```python
from build123d import *

# Parameters (mm, degrees)
F2_DEPTH = 6.35
F1_W     = 1.778
F1_H     = 3.048
F1_H_2   = 5.842
F1_W_2   = 0.762
F5_DEPTH = 12.7
F6_DEPTH = 2.54


# Not quite as in the source:
# - a feature names something its author has since deleted; it is built from what else it names


with BuildPart() as f2:
    # F0 (on Top) → F2 (new body)
    with BuildSketch(Plane.XY):
        with BuildLine():
            ThreePointArc((-19.5801208863, -2.5399817128), (-19.1839428746, -1.2973564714), (-19.05, 0))
            ThreePointArc((-19.05, 0), (-19.1839428746, 1.2973564714), (-19.5801208863, 2.5399817128))
            ThreePointArc((-19.5801208863, 2.5399817128), (-21.0323461368, 4.6093491657), (-23.1768579109, 5.9481206487))
            ThreePointArc((-23.1768579109, 5.9481206487), (-31.75, 0), (-23.1768579109, -5.9481206487))
            ThreePointArc((-23.1768579109, -5.9481206487), (-21.0323461368, -4.6093491657), (-19.5801208863, -2.5399817128))
        make_face()
        with BuildLine():
            ThreePointArc((-23.1768579109, 5.9481206487), (-21.0323461368, 4.6093491657), (-19.5801208863, 2.5399817128))
            add(Edge.make_bspline(
                [(0, 1.524), (-9.0764431036, 1.3546369813), (-12.8672626316, 1.8652065321), (-19.5801208863, 2.5399817128)],
                knots=[0, 0, 0, 0, 19.6064620154, 19.6064620154, 19.6064620154, 19.6064620154], degree=3))
            add(Edge.make_bspline(
                [(0, 1.524), (9.0764431036, 1.3546369813), (12.8672626316, 1.8652065321), (19.5801208863, 2.5399817128)],
                knots=[0, 0, 0, 0, 19.6064620154, 19.6064620154, 19.6064620154, 19.6064620154], degree=3))
            ThreePointArc((19.5801208863, 2.5399817128), (21.0323461368, 4.6093491657), (23.1768579109, 5.9481206487))
            add(Edge.make_bspline(
                [(0, 2.54), (8.1250406802, 3.246476237), (13.1090918084, 2.1852389104), (23.1768579109, 5.9481206487)],
                knots=[0, 0, 0, 0, 23.4260971776, 23.4260971776, 23.4260971776, 23.4260971776], degree=3))
            add(Edge.make_bspline(
                [(0, 2.54), (-8.1250406802, 3.246476237), (-13.1090918084, 2.1852389104), (-23.1768579109, 5.9481206487)],
                knots=[0, 0, 0, 0, 23.4260971776, 23.4260971776, 23.4260971776, 23.4260971776], degree=3))
        make_face()
        with BuildLine():
            add(Edge.make_bspline(
                [(0, -1.524), (-9.0764431036, -1.3546369813), (-12.8672626316, -1.8652065321), (-19.5801208863, -2.5399817128)],
                knots=[0, 0, 0, 0, 19.6064620154, 19.6064620154, 19.6064620154, 19.6064620154], degree=3))
            ThreePointArc((-19.5801208863, -2.5399817128), (-21.0323461368, -4.6093491657), (-23.1768579109, -5.9481206487))
            add(Edge.make_bspline(
                [(0, -2.54), (-8.1250406802, -3.246476237), (-13.1090918084, -2.1852389104), (-23.1768579109, -5.9481206487)],
                knots=[0, 0, 0, 0, 23.4260971776, 23.4260971776, 23.4260971776, 23.4260971776], degree=3))
            add(Edge.make_bspline(
                [(0, -2.54), (8.1250406802, -3.246476237), (13.1090918084, -2.1852389104), (23.1768579109, -5.9481206487)],
                knots=[0, 0, 0, 0, 23.4260971776, 23.4260971776, 23.4260971776, 23.4260971776], degree=3))
            ThreePointArc((23.1768579109, -5.9481206487), (21.0323461368, -4.6093491657), (19.5801208863, -2.5399817128))
            add(Edge.make_bspline(
                [(0, -1.524), (9.0764431036, -1.3546369813), (12.8672626316, -1.8652065321), (19.5801208863, -2.5399817128)],
                knots=[0, 0, 0, 0, 19.6064620154, 19.6064620154, 19.6064620154, 19.6064620154], degree=3))
        make_face()
        with BuildLine():
            ThreePointArc((23.1768579109, 5.9481206487), (21.0323461368, 4.6093491657), (19.5801208863, 2.5399817128))
            ThreePointArc((19.5801208863, 2.5399817128), (19.05, 0), (19.5801208863, -2.5399817128))
            ThreePointArc((19.5801208863, -2.5399817128), (21.0323461368, -4.6093491657), (23.1768579109, -5.9481206487))
            ThreePointArc((23.1768579109, -5.9481206487), (29.019775389, -5.2172527381), (31.75, 0))
            ThreePointArc((31.75, 0), (29.019775389, 5.2172527381), (23.1768579109, 5.9481206487))
        make_face()
    extrude(amount=F2_DEPTH)

    # F1 (on Front) → F3 (revolve, cut)
    with BuildSketch(Plane.XZ):
        Polygon((25.376161883, 6.35), (25.376161883, 0), (29.490961883, 0), (28.855961883, 0.635), (28.855961883, 5.715), (29.490961883, 6.35), align=None)
    revolve(axis=Axis((25.376161883, 0, 3.175), (0, 0, 1)), mode=Mode.SUBTRACT)

    # F1 (on Front) → F4 (revolve)
    with BuildSketch(Plane.XZ):
        Polygon((-22.86, 15.24), (-22.86, 12.192), (-21.844, 13.208), (-21.844, 14.224), align=None)
        with Locations((-23.749, 13.716)):
            Rectangle(F1_W, F1_H)
        with Locations((-27.051, 13.716)):
            Rectangle(F1_W, F1_H)
        Polygon((-28.956, 13.208), (-27.94, 12.192), (-27.94, 15.24), (-28.956, 14.224), align=None)
        with Locations((-27.051, 9.271)):
            Rectangle(F1_W, F1_H_2)
        with Locations((-23.749, 9.271)):
            Rectangle(F1_W, F1_H_2)
    revolve(axis=Axis((-25.4, 0, 10.795), (0, 0, 1)))

    # F1 (on Front) → F5 (cut, symmetric)
    with BuildSketch(Plane.XZ):
        with Locations((-25.019, 13.716)):
            Rectangle(F1_W_2, F1_H)
        with Locations((-25.781, 13.716)):
            Rectangle(F1_W_2, F1_H)
        with Locations((-25.019, 9.271)):
            Rectangle(F1_W_2, F1_H_2)
        with Locations((-25.781, 9.271)):
            Rectangle(F1_W_2, F1_H_2)
    extrude(amount=F5_DEPTH, both=True, mode=Mode.SUBTRACT)

    # F0 (on Top) → F6 (join)
    with BuildSketch(Plane.XY):
        with BuildLine():
            ThreePointArc((-19.5801208863, 2.5399817128), (-19.1839428746, 1.2973564714), (-19.05, 0))
            ThreePointArc((-19.05, 0), (-19.1839428746, -1.2973564714), (-19.5801208863, -2.5399817128))
            add(Edge.make_bspline(
                [(0, -1.524), (-9.0764431036, -1.3546369813), (-12.8672626316, -1.8652065321), (-19.5801208863, -2.5399817128)],
                knots=[0, 0, 0, 0, 19.6064620154, 19.6064620154, 19.6064620154, 19.6064620154], degree=3))
            add(Edge.make_bspline(
                [(0, -1.524), (9.0764431036, -1.3546369813), (12.8672626316, -1.8652065321), (19.5801208863, -2.5399817128)],
                knots=[0, 0, 0, 0, 19.6064620154, 19.6064620154, 19.6064620154, 19.6064620154], degree=3))
            ThreePointArc((19.5801208863, -2.5399817128), (19.05, 0), (19.5801208863, 2.5399817128))
            add(Edge.make_bspline(
                [(0, 1.524), (9.0764431036, 1.3546369813), (12.8672626316, 1.8652065321), (19.5801208863, 2.5399817128)],
                knots=[0, 0, 0, 0, 19.6064620154, 19.6064620154, 19.6064620154, 19.6064620154], degree=3))
            add(Edge.make_bspline(
                [(0, 1.524), (-9.0764431036, 1.3546369813), (-12.8672626316, 1.8652065321), (-19.5801208863, 2.5399817128)],
                knots=[0, 0, 0, 0, 19.6064620154, 19.6064620154, 19.6064620154, 19.6064620154], degree=3))
        make_face()
    extrude(amount=F6_DEPTH)


solid = f2.part
```
Check sheet for the modelled part. Datum: model origin and axes. Units: mm. A direction names the side the tool comes from. Coordinates: 2 decimals unless noted, no trailing zeros. Order: outer loops, then holes, each group sorted by start corner. A loop starts at its lowest first (then second) coordinate and runs counter-clockwise, first axis right, second up. Notation, with made-up numbers: (11, 64.25) -> (69, 64.25) arc R13 ccw to (69, 78.25) -> close; hole circle Ø2 at (-37, 10). An arc over 180 degrees is marked (long way). Write each question's results on one line, items separated by ' | '. Start each with the question number.
1) Set-up check for faces 1 (the face through (-21.845, -0.067, 13.723)), 2 (the face through (-28.12, 0.05, 12.37)), 3 (the face through (-28.955, 0.067, 13.723)): record each of +Z, -Z, +X, -X, +Y, -Y from which the full face is reachable in a straight line by a thin tool's end or side.
2) Draft check along Z on faces 4 (the face through (0, 0, 2.54)), 5 (the face through (-27.94, 0.05, 9.31)), 6 (the face through (-31.748, 0.171, 3.131)). Enter one of: pulls with the +Z half, pulls with the -Z half, needs draft (parallel to the pull), parting line crosses it, or undercut.
3) Material ranges on line 1 along X through (y, z) = (-0.25, 2.75); line 2 along Z through (x, y) = (10, 0.5); line 3 along Z through (x, y) = (0.5, 2.5), recorded low to high.
4) Section check A-A (z = 7). Enter the section's corners in (x, y).
5) Section check B-B (x = -25.4). Enter the section's corners in (y, z), and give its area (3 significant figures).
6) Depth check by flat-ended pin: pin 1 (2 mm diameter, centred on y = 1, z = 9, fed in from -X); pin 2 (1 mm diameter, centred on x = 11.5, z = 3, fed in from -Y); pin 3 (1.5 mm diameter, centred on x = 16.5, y = -4, fed in from +Z). Enter the tip coordinate at first touch or a pass-through.
7) Section check C-C (z = 4). Count the separate pieces of the cut face and the enclosed holes in it, and give its area (3 significant figures).
Checked values:
1) face 1: +Z, +X | face 2: -X | face 3: +Z, -X
2) face 4: pulls with the +Z half | face 5: undercut | face 6: needs draft
3) line 1: -31.75 to -19.05, 19.05 to 21.91, 28.85 to 31.75 | line 2: 0 to 2.54 | line 3: 0 to 6.35
4) outline: (-26.16, -2.42) -> (-26.16, 2.42) arc R2.54 ccw to start; (-24.64, -2.42) arc R2.54 ccw to (-24.64, 2.42) -> close
5) outline: (-6.35, 0) -> (6.35, 0) -> (6.35, 6.35) -> (-6.35, 6.35) -> close | area: 80.6 mm²
6) pin 1: x = -27.94 | pin 2: y = -3.21 | pin 3: z = 6.35
7) separate pieces: 1 | enclosed holes: 2 | area: 337 mm²
